Verification items for the finished model (mm, model axes). Face numbers are marked on the shaded views. A direction names the side the tool comes from. Coordinates: 2 decimals unless noted, no trailing zeros. Order: outer loops, then holes, each group sorted by start corner. A loop starts at its lowest first (then second) coordinate and runs counter-clockwise, first axis right, second up. Notation, with made-up numbers: M 62.25,59.5 L 88.25,59.5 A26 ccw 88.25,82.5 Z; hole C 33.25,22.25 d2. An arc over 180 degrees is marked long. Return JSON: item names as keys, results as strings. Group by question number.
1. Set-up check for the marked faces 1 and 2: record each of +Z, -Z, +X, -X, +Y, -Y from which the full face is reachable in a straight line by a thin tool's end or side.
2. Section check A-A, the plane z = -16. Record the cut outline in (x, y), plus the area to 3 significant figures.
3. Section check B-B, the plane y = 53.5. Record the cut outline in (x, z), plus the area to 3 significant figures.
4. Gauge pin test, flat ends, axial feed: pin 1 (5 mm diameter, centred on x = 132.5, y = -164, fed in from +Z); pin 2 (4.5 mm diameter, centred on y = 48, z = -27, fed in from -X); pin 3 (3 mm diameter, centred on y = -304, z = -27.5, fed in from +X). Record the tip position at first contact, or that the pin passes through.
5. Material ranges on line 1 along Y through (x, z) = (0, 2.5); line 2 along Y through (x, z) = (0, -3); line 3 along X through (y, z) = (-157, -3), recorded low to high.
6. Mould release check, pull along Y, two halves, no side actions. Record for the marked faces 3 and 4: +Y half, -Y half, draft (parallel to the pull), parting line (faces both ways), or undercut.
```python
from build123d import *

# Parameters (mm, degrees)
F1_DEPTH  = 4
F2_R      = 5.25
F2_R_2    = 90
F2_W      = 16
F2_H      = 50
F3_DEPTH  = 25
F5_DEPTH  = 30
F7_DEPTH  = 4
F8_W      = 10
F8_H      = 50
F8_R      = 5.25
F9_DEPTH  = 34.001
F10_R     = 5
F11_R     = 5
F12_DEPTH = 10
F13_W     = 15
F13_H     = 50
F14_DEPTH = 34.001


with BuildPart() as f1:
    # F0 (on Top) → F1 (new body)
    with BuildSketch(Plane.XY):
        Polygon((-424.8076211353, -344.4022295104), (0, -344.4022295104), (424.8076211353, -344.4022295104), (165, 105.5977704896), (0, 105.5977704896), (-165, 105.5977704896), align=None)
    extrude(amount=F1_DEPTH)

    # F2 (on face) → F3 (cut)
    with BuildSketch(Plane.XY.offset(4)):
        with Locations((0, -29.4022295104)):
            Circle(F2_R)
        with Locations((0, -299.4022295104)):
            Circle(F2_R)
        with Locations((-135, -164.4022295104)):
            Circle(F2_R)
        with Locations((135, -164.4022295104)):
            Circle(F2_R)
        with Locations((0, -164.4022295104)):
            Circle(F2_R_2)
        with BuildLine():
            ThreePointArc((-100, 15.5977704896), (-92, 7.5977704896), (-84, 15.5977704896))
            Line((-84, 15.5977704896), (-100, 15.5977704896))
        make_face()
        with Locations((-92, 40.5977704896)):
            Rectangle(F2_W, F2_H)
        with BuildLine():
            Line((-100, 65.5977704896), (-84, 65.5977704896))
            ThreePointArc((-84, 65.5977704896), (-92, 73.5977704896), (-100, 65.5977704896))
        make_face()
        with Locations((92, 40.5977704896)):
            Rectangle(F2_W, F2_H)
        with BuildLine():
            Line((100, 15.5977704896), (84, 15.5977704896))
            ThreePointArc((84, 15.5977704896), (92, 7.5977704896), (100, 15.5977704896))
        make_face()
        with BuildLine():
            ThreePointArc((100, 65.5977704896), (92, 73.5977704896), (84, 65.5977704896))
            Line((84, 65.5977704896), (100, 65.5977704896))
        make_face()
    extrude(amount=-F3_DEPTH, mode=Mode.SUBTRACT)

    # F4 (on face) → F5 (join)
    with BuildSketch(Plane(origin=(0, 0, 0), x_dir=(1, 0, 0), z_dir=(0, 0, -1))):
        Polygon((-161.5358983849, -103.5977704896), (-165, -105.5977704896), (165, -105.5977704896), (161.5358983849, -103.5977704896), (162.6905989232, -101.5977704896), (-162.6905989232, -101.5977704896), align=None)
        Polygon((-422.4982200586, 340.4022295104), (-165, -105.5977704896), (-165, -101.5977704896), (-162.6905989232, -101.5977704896), (-417.8794179051, 340.4022295104), align=None)
        Polygon((-165, -101.5977704896), (-165, -105.5977704896), (-161.5358983849, -103.5977704896), (-162.6905989232, -101.5977704896), align=None)
        Polygon((161.5358983849, -103.5977704896), (165, -105.5977704896), (165, -101.5977704896), (162.6905989232, -101.5977704896), align=None)
        Polygon((165, -101.5977704896), (165, -105.5977704896), (422.4982200586, 340.4022295104), (417.8794179051, 340.4022295104), (162.6905989232, -101.5977704896), align=None)
        Polygon((-423.652920597, 342.4022295104), (-422.4982200586, 340.4022295104), (-417.8794179051, 340.4022295104), (-420.1888189818, 344.4022295104), align=None)
        Polygon((417.8794179051, 340.4022295104), (422.4982200586, 340.4022295104), (424.8076211353, 344.4022295104), (420.1888189818, 344.4022295104), align=None)
        Polygon((-420.1888189818, 344.4022295104), (-417.8794179051, 340.4022295104), (417.8794179051, 340.4022295104), (420.1888189818, 344.4022295104), align=None)
        Polygon((-424.8076211353, 344.4022295104), (-423.652920597, 342.4022295104), (-420.1888189818, 344.4022295104), align=None)
    extrude(amount=F5_DEPTH)

    # F6 (on face) → F7 (join)
    with BuildSketch(Plane(origin=(0, 0, -30), x_dir=(1, 0, 0), z_dir=(0, 0, -1))):
        Polygon((-424.8076211353, 344.4022295104), (-476.7691453624, 314.4022295104), (-234.2820323028, -105.5977704896), (-182.3205080757, -75.5977704896), align=None)
        Polygon((234.2820323028, -105.5977704896), (476.7691453624, 314.4022295104), (424.8076211353, 344.4022295104), (182.3205080757, -75.5977704896), align=None)
    extrude(amount=-F7_DEPTH)

    # F8 (on face) → F9 (cut, through all)
    with BuildSketch(Plane(origin=(0, 0, -30), x_dir=(1, 0, 0), z_dir=(0, 0, -1))):
        with BuildLine():
            ThreePointArc((-240, -75.5977704896), (-235, -80.5977704896), (-230, -75.5977704896))
            Line((-230, -75.5977704896), (-240, -75.5977704896))
        make_face()
        with Locations((-235, -50.5977704896)):
            Rectangle(F8_W, F8_H)
        with BuildLine():
            Line((-240, -25.5977704896), (-230, -25.5977704896))
            ThreePointArc((-230, -25.5977704896), (-235, -20.5977704896), (-240, -25.5977704896))
        make_face()
        with Locations((0, 29.4022295104)):
            Circle(F8_R)
        with BuildLine():
            ThreePointArc((-290, 11.0047698888), (-285, 6.0047698888), (-280, 11.0047698888))
            Line((-280, 11.0047698888), (-280, 61.0047698888))
            ThreePointArc((-280, 61.0047698888), (-285, 66.0047698888), (-290, 61.0047698888))
            Line((-290, 61.0047698888), (-290, 11.0047698888))
        make_face()
        with BuildLine():
            ThreePointArc((-340, 97.6073102673), (-335, 92.6073102673), (-330, 97.6073102673))
            Line((-330, 97.6073102673), (-330, 147.6073102673))
            ThreePointArc((-330, 147.6073102673), (-335, 152.6073102673), (-340, 147.6073102673))
            Line((-340, 147.6073102673), (-340, 97.6073102673))
        make_face()
        with BuildLine():
            ThreePointArc((-390, 184.2098506457), (-385, 179.2098506457), (-380, 184.2098506457))
            Line((-380, 184.2098506457), (-380, 234.2098506457))
            ThreePointArc((-380, 234.2098506457), (-385, 239.2098506457), (-390, 234.2098506457))
            Line((-390, 234.2098506457), (-390, 184.2098506457))
        make_face()
        with BuildLine():
            ThreePointArc((-440, 270.8123910242), (-435, 265.8123910242), (-430, 270.8123910242))
            Line((-430, 270.8123910242), (-430, 320.8123910242))
            ThreePointArc((-430, 320.8123910242), (-435, 325.8123910242), (-440, 320.8123910242))
            Line((-440, 320.8123910242), (-440, 270.8123910242))
        make_face()
        with BuildLine():
            ThreePointArc((380, 184.2098506457), (385, 179.2098506457), (390, 184.2098506457))
            Line((390, 184.2098506457), (390, 234.2098506457))
            ThreePointArc((390, 234.2098506457), (385, 239.2098506457), (380, 234.2098506457))
            Line((380, 234.2098506457), (380, 184.2098506457))
        make_face()
        with BuildLine():
            ThreePointArc((430, 270.8123910242), (435, 265.8123910242), (440, 270.8123910242))
            Line((440, 270.8123910242), (440, 320.8123910242))
            ThreePointArc((440, 320.8123910242), (435, 325.8123910242), (430, 320.8123910242))
            Line((430, 320.8123910242), (430, 270.8123910242))
        make_face()
        with BuildLine():
            ThreePointArc((340, 147.6073102673), (335, 152.6073102673), (330, 147.6073102673))
            Line((330, 147.6073102673), (330, 97.6073102673))
            ThreePointArc((330, 97.6073102673), (335, 92.6073102673), (340, 97.6073102673))
            Line((340, 97.6073102673), (340, 147.6073102673))
        make_face()
        with Locations((235, -50.5977704896)):
            Rectangle(F8_W, F8_H)
        with BuildLine():
            Line((240, -75.5977704896), (230, -75.5977704896))
            ThreePointArc((230, -75.5977704896), (235, -80.5977704896), (240, -75.5977704896))
        make_face()
        with BuildLine():
            ThreePointArc((240, -25.5977704896), (235, -20.5977704896), (230, -25.5977704896))
            Line((230, -25.5977704896), (240, -25.5977704896))
        make_face()
        with BuildLine():
            ThreePointArc((280, 11.0047698888), (285, 6.0047698888), (290, 11.0047698888))
            Line((290, 11.0047698888), (290, 61.0047698888))
            ThreePointArc((290, 61.0047698888), (285, 66.0047698888), (280, 61.0047698888))
            Line((280, 61.0047698888), (280, 11.0047698888))
        make_face()
    extrude(amount=-F9_DEPTH, mode=Mode.SUBTRACT)

    # F10
    f10_edges = [f1.edges().sort_by_distance(p)[0] for p in [
        (-476.769145, -314.40223, -28),
        (-234.282032, 105.59777, -28),
        (234.282032, 105.59777, -28),
        (476.769145, -314.40223, -28),
    ]]
    fillet(f10_edges, radius=F10_R)

    # F11 (on face) → F12 (join)
    with BuildSketch(Plane(origin=(0, 0, 0), x_dir=(1, 0, 0), z_dir=(0, 0, -1))):
        Polygon((-135, 154.5872749342), (-126.5, 159.4947522223), (-126.5, 169.3097067985), (-135, 174.2171840866), (-143.5, 169.3097067985), (-143.5, 159.4947522223), align=None)
        with Locations((-135, 164.4022295104)):
            Circle(F11_R, mode=Mode.SUBTRACT)
        Polygon((126.5, 159.4947522223), (135, 154.5872749342), (143.5, 159.4947522223), (143.5, 169.3097067985), (135, 174.2171840866), (126.5, 169.3097067985), align=None)
        with Locations((135, 164.4022295104)):
            Circle(F11_R, mode=Mode.SUBTRACT)
        Polygon((-8.5, 294.4947522223), (0, 289.5872749342), (8.5, 294.4947522223), (8.5, 304.3097067985), (0, 309.2171840866), (-8.5, 304.3097067985), align=None)
        with Locations((0, 299.4022295104)):
            Circle(F11_R, mode=Mode.SUBTRACT)
        Polygon((0, 19.5872749342), (8.5, 24.4947522223), (8.5, 34.3097067985), (0, 39.2171840866), (-8.5, 34.3097067985), (-8.5, 24.4947522223), align=None)
        with Locations((0, 29.4022295104)):
            Circle(F11_R, mode=Mode.SUBTRACT)
    extrude(amount=F12_DEPTH)

    # F13 (on face) → F14 (cut, through all)
    with BuildSketch(Plane.XY.offset(4)):
        with BuildLine():
            ThreePointArc((-149, -319.4022295104), (-141.5, -326.9022295104), (-134, -319.4022295104))
            Line((-134, -319.4022295104), (-149, -319.4022295104))
        make_face()
        with Locations((-141.5, -294.4022295104)):
            Rectangle(F13_W, F13_H)
        with BuildLine():
            Line((-149, -269.4022295104), (-134, -269.4022295104))
            ThreePointArc((-134, -269.4022295104), (-141.5, -261.9022295104), (-149, -269.4022295104))
        make_face()
        with BuildLine():
            ThreePointArc((149, -269.4022295104), (141.5, -261.9022295104), (134, -269.4022295104))
            Line((134, -269.4022295104), (134, -319.4022295104))
            ThreePointArc((134, -319.4022295104), (141.5, -326.9022295104), (149, -319.4022295104))
            Line((149, -319.4022295104), (149, -269.4022295104))
        make_face()
    extrude(amount=-F14_DEPTH, mode=Mode.SUBTRACT)


solid = f1.part
```
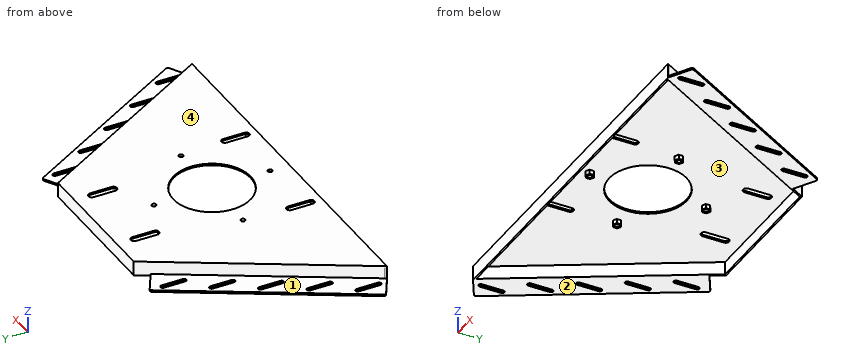
Answers follow:
{
 "1": {"face 1": "+Z, -X, +Y", "face 2": "-Z, +X, -X, +Y, -Y"},
 "2": {"outline": "M -424.81,-344.4 L 424.81,-344.4 L 165,105.6 L -165,105.6 Z; hole M -417.88,-340.4 L 417.88,-340.4 L 162.69,101.6 L -162.69,101.6 Z", "area": "8,800 mm^2"},
 "3": {"outline": "M -264.36,-30 L -240,-30 L -240,-26 L -264.36,-26 Z; M -230,-30 L -190.46,-30 L -190.46,0 L -100,0 L -100,4 L -195.08,4 L -195.08,-26 L -230,-26 Z; M -84,0 L 84,0 L 84,4 L -84,4 Z; M 100,0 L 190.46,0 L 190.46,-30 L 230,-30 L 230,-26 L 195.08,-26 L 195.08,4 L 100,4 Z; M 240,-30 L 264.36,-30 L 264.36,-26 L 240,-26 Z", "area": "2,180 mm^2"},
 "4": {"pin 1": "z = 0", "pin 2": "x = -268.84", "pin 3": "x = 471.63"},
 "5": {"line 1": "-344.4 to -304.65, -294.15 to -254.4, -74.4 to -34.65, -24.15 to 105.6", "line 2": "-344.4 to -340.4, -309.22 to -304.4, -294.4 to -289.59, -39.22 to -34.4, -24.4 to -19.59, 101.6 to 105.6", "line 3": "-316.61 to -311.99, -139.18 to -130.82, 130.82 to 139.18, 311.99 to 316.61"},
 "6": {"face 3": "undercut", "face 4": "draft"}
}
